from build123d import *

# Parameters (mm, degrees)
SKETCH1_R           = 70
BOSS_EXTRUDE1_DEPTH = 11
SKETCH2_R           = 12.5
CUT_EXTRUDE1_DEPTH  = 100.604216778
SKETCH3_R           = 7.874590161
CUT_EXTRUDE2_DEPTH  = 10.562321
CIRPATTERN1_START   = 0.437678763
CIRPATTERN1_DEPTH   = 10.562321237


# Read off the part's stored shape, not the designer's step: CirPattern1
with BuildPart() as part:
    # Sketch1 → Boss-Extrude1 (new body)
    with BuildSketch(Plane(origin=(0, 0, 0), x_dir=(1, 0, 0), z_dir=(0, 1, 0))):
        with Locations(Location((0, 0, 0), (0, 0, 270))):
            Circle(SKETCH1_R)
    extrude(amount=BOSS_EXTRUDE1_DEPTH)

    # Sketch2 → Cut-Extrude1 (cut, through all)
    with BuildSketch(Plane(origin=(0, 0, 0), x_dir=(1, 0, 0), z_dir=(0, 1, 0))):
        with Locations(Location((0, 0, 0), (0, 0, 270))):
            Circle(SKETCH2_R)
    extrude(amount=CUT_EXTRUDE1_DEPTH, mode=Mode.SUBTRACT)

    # Sketch3 → Cut-Extrude2 (cut)
    with BuildSketch(Plane(origin=(0, 11, 0), x_dir=(1, 0, 0), z_dir=(0, 1, 0))):
        with Locations((-11.334309292, 0)):
            Circle(SKETCH3_R)
    extrude(amount=-CUT_EXTRUDE2_DEPTH, mode=Mode.SUBTRACT)

    # CirPattern1 outline → CirPattern1 (cut)
    with BuildSketch(Plane(origin=(0, 0, 0), x_dir=(1, 0, 0), z_dir=(0, 1, 0)).offset(CIRPATTERN1_START)):
        with BuildLine():
            ThreePointArc((-9.82448031, -7.728491874), (-11.53482537, -7.872036808), (-13.235644462, -7.641602893))
            ThreePointArc((-13.235644462, -7.641602893), (-9.604449727, -16.635394905), (0, -15.283205786))
            ThreePointArc((0, -15.283205786), (9.604449727, -16.635394905), (13.235644462, -7.641602893))
            ThreePointArc((13.235644462, -7.641602893), (19.208899453, 0), (13.235644462, 7.641602893))
            ThreePointArc((13.235644462, 7.641602893), (9.604449727, 16.635394905), (0, 15.283205786))
            ThreePointArc((0, 15.283205786), (-9.604449727, 16.635394905), (-13.235644462, 7.641602893))
            ThreePointArc((-13.235644462, 7.641602893), (-11.53482537, 7.872036808), (-9.82448031, 7.728491874))
            ThreePointArc((-9.82448031, 7.728491874), (12.5, 0), (-9.82448031, -7.728491874))
        make_face()
    extrude(amount=CIRPATTERN1_DEPTH, mode=Mode.SUBTRACT)


solid = part.part
Can you work these out from the model? Positions are in its coordinate system, mm. A direction names the side the tool comes from. Coordinates: 2 decimals unless noted, no trailing zeros. Loops run counter-clockwise (first coordinate to the right, second up) from the corner with the lowest first, then second, coordinate; pieces in that order, holes last. Notation, with made-up numbers: (41.25, -25) - (88.25, -25) arc R12 cw to (88.25, -19) - close; hole circle Ø7 at (-35.75, 20.5). An arc over 180 degrees is marked (long way). Answer as a JSON object with one key per item and string values. Group by question number.
Item 1: If we section it at D-D (z = -53): List the corners of the cut face in (x, y) for me, plus the area to 3 significant figures.
Item 2: For pin 1 (15 mm diameter, centred on x = 0, z = 0, fed in from +Y); pin 2 (1.5 mm diameter, centred on y = 7.5, z = -48, fed in from -X); pin 3 (1.5 mm diameter, centred on y = 8.5, z = -14, fed in from -X); pin 4 (2 mm diameter, centred on y = 9, z = 0.5, fed in from +X), each with a flat end and sliding along its axis, tell me the tip position at first contact or that it passes through.
Item 3: If we mould it in two halves opening along X, with no side actions, what happens to faces 3 (the face through (1, 11, -17)), 4 (the face through (3.755, 0.216, 11.923)), 5 (the face through (-42.594, 5.423, -55.55))? For each: released by +X, released by -X, zero draft, split by the parting line, or undercut.
Item 4: If we section it at C-C (x = -21.5): List the corners of the cut face in (y, z) for me, plus the area to 3 significant figures.
Item 5: If I drill on L1, parallel to X at y = 0.35, z = 0; L2, parallel to X at y = 9.5, z = -16; L3, parallel to Z at x = 10.5, y = 7.75, over which ranges is the centre line in solid material (lowest first)? Write a range as from..to.
Item 6: If we section it at B-B (x = -4): List the corners of the cut face in (y, z) for me, plus the area to 3 significant figures.
Item 7: If we section it at A-A (z = 0): List the corners of the cut face in (x, y) for me, plus the area to 3 significant figures.
Item 8: On a 3-axis mill with a long thin cutter (end or side, diameter ignored), from which of +Z, -Z, +X, -X, +Y, -Y can I reach the whole of each face in a straight line? I mean faces 1 (the face through (9.477, 5.645, 16.707)), 2 (the face through (-15, 0, -1)). Say none if no direction works.
Returned:
{
 "1": {"outline": "(-45.73, 0) - (45.73, 0) - (45.73, 11) - (-45.73, 11) - close", "area": "1,010 mm²"},
 "2": {"pin 1": "passes through", "pin 2": "stops at x = -51.65", "pin 3": "stops at x = -68.73", "pin 4": "stops at x = 70"},
 "3": {"face 3": "zero draft", "face 4": "undercut", "face 5": "split by the parting line"},
 "4": {"outline": "(0, -66.62) - (11, -66.62) - (11, 66.62) - (0, 66.62) - close", "area": "1,470 mm²"},
 "5": {"L1": "x = -70..-12.5, 12.5..70", "L2": "x = -68.15..-10.54, -0.79..0.79, 10.54..68.15", "L3": "z = -69.21..-16.03, 16.03..69.21"},
 "6": {"outline": "(0, -69.89) - (11, -69.89) - (11, -17.51) - (0.44, -17.51) - (0.44, -11.84) - (0, -11.84) - close; (0, 11.84) - (0.44, 11.84) - (0.44, 17.51) - (11, 17.51) - (11, 69.89) - (0, 69.89) - close", "area": "1,160 mm²"},
 "7": {"outline": "(-70, 0) - (-12.5, 0) - (-12.5, 0.44) - (-19.21, 0.44) - (-19.21, 11) - (-70, 11) - close; (12.5, 0) - (70, 0) - (70, 11) - (19.21, 11) - (19.21, 0.44) - (12.5, 0.44) - close", "area": "1,120 mm²"},
 "8": {"face 1": "+Y", "face 2": "+Z, -Z, +X, -X, -Y"}
}
